```python
from build123d import *

# Parameters (mm, degrees)
ESTRUSIONE_ESTRUSIONE2_DEPTH = 1.6
SCHIZZO2_R                   = 2
TAGLIO_ESTRUSIONE1_DEPTH     = 10
SCHIZZO8_W                   = 53.4
SCHIZZO8_H                   = 21.2
SCHIZZO8_W_2                 = 6.4
SCHIZZO8_H_2                 = 21.96
SCHIZZO8_W_3                 = 38
SCHIZZO8_H_3                 = 12
ESTRUSIONE_ESTRUSIONE3_DEPTH = 10
FORO_3_1_3_1_1_D             = 3.1
SCHIZZO12_W                  = 12
SCHIZZO12_H                  = 16
TAGLIO_ESTRUSIONE2_DEPTH     = 10


with BuildPart() as part:
    # bordo2 → Estrusione-Estrusione2 (new body)
    with BuildSketch(Plane.XY):
        with BuildLine():
            Line((-158.754433684, 116.187089821), (-158.754433684, -3.865947122))
            ThreePointArc((-158.754433684, -3.865947122), (-156.505538032, -9.426954116), (-151.023233988, -11.861429997))
            Line((-151.023233988, -11.861429997), (-16.437702381, -16.386063763))
            ThreePointArc((-16.437702381, -16.386063763), (-13.471762347, -16.861957987), (-10.716938169, -18.059546957))
            ThreePointArc((-10.716938169, -18.059546957), (0.214142299, -20.99890814), (11.083005754, -17.837235869))
            ThreePointArc((11.083005754, -17.837235869), (13.822228864, -16.580762318), (16.788120425, -16.046387663))
            Line((16.788120425, -16.046387663), (113.64611863, -10.970275071))
            ThreePointArc((113.64611863, -10.970275071), (115.127499694, -11.516785399), (115.750790543, -12.967534141))
            Line((115.750790543, -12.967534141), (115.750790543, -13.091597346))
            ThreePointArc((115.750790543, -13.091597346), (116.336576981, -14.505810909), (117.750790543, -15.091597346))
            Line((117.750790543, -15.091597346), (193, -15.091597346))
            ThreePointArc((193, -15.091597346), (198.656854249, -12.748451596), (201, -7.091597346))
            Line((201, -7.091597346), (201, -2.727936118))
            ThreePointArc((201, -2.727936118), (206.640455622, 14.782420751), (221.440839847, 25.708351564))
            Line((221.440839847, 25.708351564), (247.399963271, 34.43478664))
            ThreePointArc((247.399963271, 34.43478664), (271.481734612, 52.716367083), (280.623213556, 81.536173764))
            Line((280.623213556, 81.536173764), (280.623213556, 120.714334058))
            ThreePointArc((280.623213556, 120.714334058), (278.556224626, 129.569113216), (272.782502161, 136.593619325))
            ThreePointArc((272.782502161, 136.593619325), (236.38547949, 150.641341579), (198.16455661, 142.815562768))
            ThreePointArc((198.16455661, 142.815562768), (186.818545747, 138.475666611), (174.760806771, 137))
            Line((174.760806771, 137), (124.67436916, 137))
            ThreePointArc((124.67436916, 137), (119.429676247, 137.580068398), (114.43850672, 139.292233645))
            ThreePointArc((114.43850672, 139.292233645), (106.197691209, 138.475942424), (103.023486693, 130.82729566))
            ThreePointArc((103.023486693, 130.82729566), (102.639348768, 125.614781735), (100.075807145, 121.059991103))
            ThreePointArc((100.075807145, 121.059991103), (99.881158934, 120.843862569), (99.686086367, 120.628116972))
            ThreePointArc((99.686086367, 120.628116972), (98.127896826, 119.187643435), (96.340342687, 118.044153663))
            ThreePointArc((96.340342687, 118.044153663), (90.73314925, 115.468824104), (84.896818522, 113.466279669))
            ThreePointArc((84.896818522, 113.466279669), (81.223809571, 111.391901357), (78.878619087, 107.885603918))
            ThreePointArc((78.878619087, 107.885603918), (76.807046099, 105.140996793), (73.568687614, 103.984572456))
            Line((73.568687614, 103.984572456), (47.908191181, 102.639762823))
            ThreePointArc((47.908191181, 102.639762823), (39.500299817, 103.697237213), (31.984038936, 107.610894282))
            ThreePointArc((31.984038936, 107.610894282), (27.325075003, 108.10748534), (24.779841609, 104.173742266))
            ThreePointArc((24.779841609, 104.173742266), (23.153545862, 102.254723235), (20.936931048, 103.443878677))
            ThreePointArc((20.936931048, 103.443878677), (11.600258518, 111.566065701), (-0.535174134, 109.142297901))
            ThreePointArc((-0.535174134, 109.142297901), (-3.341686704, 107.964824618), (-6.364881252, 108.315895646))
            ThreePointArc((-6.364881252, 108.315895646), (-9.502789582, 108.987631441), (-12.691899138, 108.630871146))
            ThreePointArc((-12.691899138, 108.630871146), (-20.24385632, 107.770369186), (-27.692371148, 109.284353259))
            ThreePointArc((-27.692371148, 109.284353259), (-30.106556798, 111.496306745), (-30.999967426, 114.646361987))
            Line((-30.999967426, 114.646361987), (-30.999963226, 116.187057109))
            ThreePointArc((-30.999963226, 116.187057109), (-36.980182385, 126.620513133), (-49, 127))
            ThreePointArc((-49, 127), (-52.072194014, 124.94805369), (-54.892871514, 122.562128679))
            ThreePointArc((-54.892871514, 122.562128679), (-63.960512309, 119.217688785), (-72.552773096, 123.642668149))
            ThreePointArc((-72.552773096, 123.642668149), (-75.205541561, 126.063997519), (-78.456042527, 127.591826018))
            ThreePointArc((-78.456042527, 127.591826018), (-78.680837, 127.65808008), (-78.905966578, 127.72318637))
            ThreePointArc((-78.905966578, 127.72318637), (-80.541919682, 128.070548042), (-82.210278367, 128.187089821))
            Line((-82.210278367, 128.187089821), (-146.754433684, 128.187089821))
            ThreePointArc((-146.754433684, 128.187089821), (-155.239715059, 124.672371195), (-158.754433684, 116.187089821))
        make_face()
    extrude(amount=ESTRUSIONE_ESTRUSIONE2_DEPTH)

    # Schizzo2 → Taglio-Estrusione1 (cut)
    with BuildSketch(Plane.XY.offset(1.6)):
        with Locations((110.578126436, 84.562458849)):
            Circle(SCHIZZO2_R)
        with Locations((184, 45)):
            Circle(SCHIZZO2_R)
        with Locations((-115.131933684, 84.277035982)):
            Circle(SCHIZZO2_R)
        with Locations((-115.131933684, 109.187589821)):
            Circle(SCHIZZO2_R)
    extrude(amount=-TAGLIO_ESTRUSIONE1_DEPTH, mode=Mode.SUBTRACT)

    # Schizzo8 → Estrusione-Estrusione3 (add)
    with BuildSketch(Plane.XY):
        with Locations((145.200028088, 122.829953321)):
            Rectangle(SCHIZZO8_W, SCHIZZO8_H)
        with Locations((-144.999971912, 114.999953321)):
            Rectangle(SCHIZZO8_W_2, SCHIZZO8_H_2)
        with Locations((187.245628088, 118.999953321)):
            Rectangle(SCHIZZO8_W_2, SCHIZZO8_H_2)
        with Locations((-54.041371912, 107.999953321)):
            Rectangle(SCHIZZO8_W_3, SCHIZZO8_H_3)
    extrude(amount=ESTRUSIONE_ESTRUSIONE3_DEPTH)

    # Foro Ø3.1 (3.1)-1 (through all)
    with Locations(Plane.XY.offset(1.6)):
        with Locations((-105.606713702, 123.757761503), (-150.881154472, 74.423504607), (-148.705373273, -7.765150729), (0, -17.434580106), (0, 20.969513485), (-0.120683654, 70.999897433), (98.633890728, 109.736207798), (197.634129984, 68.336031239), (194.042729825, -6.748739049), (113.891576714, -3.672362968), (270.790603772, 105.604483849), (197.521931264, 134.344122063)):
            Hole(FORO_3_1_3_1_1_D / 2)

    # Schizzo12 → Taglio-Estrusione2 (cut)
    with BuildSketch(Plane.XY.offset(1.6)):
        with Locations((230.408257616, 80.165324897)):
            Rectangle(SCHIZZO12_W, SCHIZZO12_H)
    extrude(amount=-TAGLIO_ESTRUSIONE2_DEPTH, mode=Mode.SUBTRACT)


solid = part.part
```
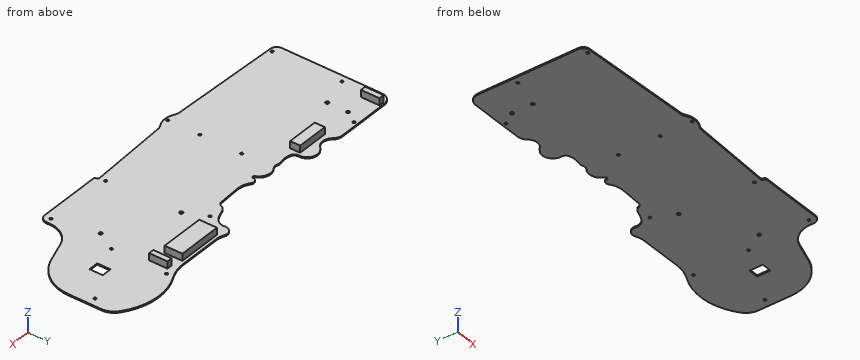
CAD build for the part. Positions are in the model's coordinates, mm. Give positions to 0.01 mm unless a question says otherwise; leave off trailing zeros. Write each loop counter-clockwise with the first axis right and the second up, starting at its lowest first coordinate (ties: lowest second). Pieces come first, ordered by that corner, then holes. Notation, with made-up numbers: (1, 67) -> (24, 67) arc R22 cw to (24, 97) -> close; hole circle Ø2 at (-14.75, -17.5). An arc over 180 degrees is marked (long way). Write each question's results on one line, items separated by ' | '.
1. Cut at C-C, the plane x = -21. Write the cut outline in (y, z).
Geometry check:
outline: (-16.23, 0) -> (107.82, 0) -> (107.82, 1.6) -> (-16.23, 1.6) -> close
2. Wall check: probe 1 along X at (y, z) = (117, 6); probe 2 along X at (y, z) = (127, 8.5); probe 3 along Y at (x, z) = (0, 0.8). Give the ranges that are in metal, low to high. Write a range as [from, to].
Geometry check:
probe 1: [-148.2, -141.8], [118.5, 171.9], [184.05, 190.45] | probe 2: [118.5, 171.9], [184.05, 190.45] | probe 3: [-21, -18.98], [-15.88, 19.42], [22.52, 69.45], [72.55, 109.53]
3. Cut at B-B, the plane y = 94. Write the cut outline in (x, z).
Geometry check:
outline: (-158.75, 0) -> (280.62, 0) -> (280.62, 1.6) -> (-158.75, 1.6) -> close
4. Drop flat-ended pins along their axis: P1, Ø8, axis at x = 58, y = 46, coming from the +Z side; P2, Ø0.5, axis at x = 160.5, z = 0.5, coming from the +Y side; P3, Ø2.5, axis at y = 116, z = 5, coming from the +X side. Give the stop position or say it passes through.
Geometry check:
P1: z = 1.6 | P2: y = 137 | P3: x = 190.45
5. Cut at A-A, the plane z = 3.5. Write the cut outline in (x, y).
Geometry check:
outline: (-148.2, 104.02) -> (-141.8, 104.02) -> (-141.8, 125.98) -> (-148.2, 125.98) -> close; (-73.04, 102) -> (-35.04, 102) -> (-35.04, 114) -> (-73.04, 114) -> close; (118.5, 112.23) -> (171.9, 112.23) -> (171.9, 133.43) -> (118.5, 133.43) -> close; (184.05, 108.02) -> (190.45, 108.02) -> (190.45, 129.98) -> (184.05, 129.98) -> close
